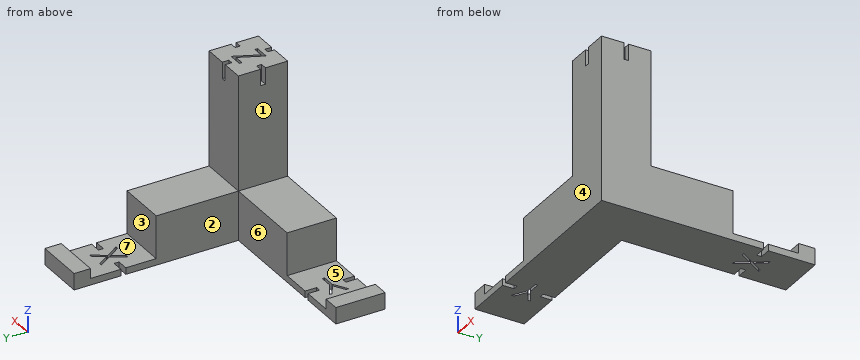
from build123d import *

# Parameters (mm, degrees)
CROQUIS2_W                = 25
CROQUIS2_H                = 15
SALIENTE_EXTRUIR1_DEPTH   = 15
CROQUIS2_W_2              = 15
CROQUIS2_H_2              = 25
SALIENTE_EXTRUIR1_2_DEPTH = 15
CROQUIS2_3_W              = 15
CROQUIS2_3_H              = 15
SALIENTE_EXTRUIR2_DEPTH   = 50
CROQUIS3_W                = 20
CROQUIS3_H                = 15
CROQUIS3_W_2              = 15
CROQUIS3_H_2              = 20
SALIENTE_EXTRUIR3_DEPTH   = 2
CROQUIS3_3_W              = 5
CROQUIS3_3_H              = 15
CROQUIS3_3_W_2            = 15
CROQUIS3_3_H_2            = 5
SALIENTE_EXTRUIR4_DEPTH   = 5
CROQUIS4_W                = 3.5
CROQUIS4_H                = 1.5
CROQUIS4_W_2              = 1.5
CROQUIS4_H_2              = 3.5
CORTAR_EXTRUIR1_DEPTH     = 15
CROQUIS5_W                = 1.5
CROQUIS5_H                = 2
CROQUIS5_W_2              = 2
CROQUIS5_H_2              = 1.5
CORTAR_EXTRUIR2_DEPTH     = 5


with BuildPart() as part:
    # Croquis2 → Saliente-Extruir1 (new body)
    with BuildSketch(Plane.XY):
        with Locations((-27.5, 7.5)):
            Rectangle(CROQUIS2_W, CROQUIS2_H)
    extrude(amount=SALIENTE_EXTRUIR1_DEPTH)



with BuildPart() as body_2:
    # Croquis2 → Saliente-Extruir1 2 (new body)
    with BuildSketch(Plane.XY):
        with Locations((-7.5, 27.5)):
            Rectangle(CROQUIS2_W_2, CROQUIS2_H_2)
    extrude(amount=SALIENTE_EXTRUIR1_2_DEPTH)


with BuildPart() as part_1:
    add(part.part)

    add(body_2.part)  # Saliente-Extruir2 merges body 2
    # Croquis2_3 → Saliente-Extruir2 (add)
    with BuildSketch(Plane.XY):
        with Locations((-7.5, 7.5)):
            Rectangle(CROQUIS2_3_W, CROQUIS2_3_H)
    extrude(amount=SALIENTE_EXTRUIR2_DEPTH)

    # Croquis3 → Saliente-Extruir3 (add)
    with BuildSketch(Plane.XY):
        with Locations((-50, 7.5)):
            Rectangle(CROQUIS3_W, CROQUIS3_H)
        with Locations((-7.5, 50)):
            Rectangle(CROQUIS3_W_2, CROQUIS3_H_2)
    extrude(amount=SALIENTE_EXTRUIR3_DEPTH)

    # Croquis3_3 → Saliente-Extruir4 (add)
    with BuildSketch(Plane.XY):
        with Locations((-62.5, 7.5)):
            Rectangle(CROQUIS3_3_W, CROQUIS3_3_H)
        with Locations((-7.5, 62.5)):
            Rectangle(CROQUIS3_3_W_2, CROQUIS3_3_H_2)
    extrude(amount=SALIENTE_EXTRUIR4_DEPTH)

    # Croquis4 → Cortar-Extruir1 (cut)
    with BuildSketch(Plane.XY.offset(2)):
        with Locations((-13.25, 50)):
            Rectangle(CROQUIS4_W, CROQUIS4_H)
        with Locations((-1.75, 50)):
            Rectangle(CROQUIS4_W, CROQUIS4_H)
        with Locations((-50, 13.25)):
            Rectangle(CROQUIS4_W_2, CROQUIS4_H_2)
        with Locations((-50, 1.75)):
            Rectangle(CROQUIS4_W_2, CROQUIS4_H_2)
        Polygon((-10.423076923, 54), (-9.594551282, 54), (-7.5, 50.727564103), (-5.405448718, 54), (-4.576923077, 54), (-7.084935897, 50.080128205), (-4.474358974, 46), (-5.302884615, 46), (-7.5, 49.432692308), (-9.697115385, 46), (-10.525641026, 46), (-7.913461538, 50.080128205), align=None)
        Polygon((-54, 10.423076923), (-54, 9.600961538), (-50.5625, 7.498397436), (-54, 5.399038462), (-54, 4.576923077), (-49.802884615, 7.141025641), (-46, 7.141025641), (-46, 7.858974359), (-49.802884615, 7.858974359), align=None)
    extrude(amount=-CORTAR_EXTRUIR1_DEPTH, mode=Mode.SUBTRACT)

    # Croquis5 → Cortar-Extruir2 (cut)
    with BuildSketch(Plane.XY.offset(50)):
        with Locations((-7.5, 14)):
            Rectangle(CROQUIS5_W, CROQUIS5_H)
        with Locations((-7.5, 1)):
            Rectangle(CROQUIS5_W, CROQUIS5_H)
        with Locations((-1, 7.5)):
            Rectangle(CROQUIS5_W_2, CROQUIS5_H_2)
        with Locations((-14, 7.5)):
            Rectangle(CROQUIS5_W_2, CROQUIS5_H_2)
        Polygon((-9.551282051, 10.679487179), (-9.551282051, 11.5), (-5.346153846, 11.5), (-8.701923077, 4.320512821), (-5.448717949, 4.320512821), (-5.448717949, 3.5), (-9.858974359, 3.5), (-6.503205128, 10.679487179), align=None)
    extrude(amount=-CORTAR_EXTRUIR2_DEPTH, mode=Mode.SUBTRACT)


solid = part_1.part
Could you check a few things on this model? Use its own coordinates, in mm. Face numbers are marked on the shaded views. A direction names the side the tool comes from. Give positions to 0.01 mm unless a question says otherwise; leave off trailing zeros. Order: outer loops, then holes, each group sorted by start corner. A loop starts at its lowest first (then second) coordinate and runs counter-clockwise, first axis right, second up.
1. Suppose I cut it at C-C (z = 14). Write out the boundary of the cut face in (x, y), plus the area to 3 significant figures.
Answers below:
outline: (-40, 0) - (0, 0) - (0, 40) - (-15, 40) - (-15, 15) - (-40, 15) - close
area: 975 mm2
2. I need wall thicknesses on L1, parallel to X at y = 36, z = 11; L2, parallel to X at y = 9.5, z = 12.5; L3, parallel to Z at x = -16.5, y = 6. Which ranges of each line are inside material? Lowest first, please.
Answers below:
L1: x = -15 to 0
L2: x = -40 to 0
L3: z = 0 to 15
3. Thinking about a two-plate mould opening in Y: for the marked faces 4, 5, 6 and 7, which applies, +Y half, -Y half, draft (parallel to the pull), parting line (faces both ways), or undercut?
Answers below:
face 4: -Y half
face 5: draft
face 6: +Y half
face 7: undercut
4. Suppose I cut it at B-B (y = 47.5). Write out the boundary of the cut face in (x, z), plus the area to 3 significant figures.
Answers below:
outline: (-15, 0) - (-9.57, 0) - (-9.57, 2) - (-15, 2) - close; (-8.74, 0) - (-6.26, 0) - (-6.26, 2) - (-8.74, 2) - close; (-5.43, 0) - (0, 0) - (0, 2) - (-5.43, 2) - close
area: 26.7 mm2
5. Suppose I cut it at D-D (y = 19). Write out the boundary of the cut face in (x, z).
Answers below:
outline: (-15, 0) - (0, 0) - (0, 15) - (-15, 15) - close
6. Which directions (+Z, -Z, +X, -X, +Y, -Y) give clear straight access to the entire face, cutting with the end or side of a thin tool? Please do the marked faces 1, 2 and 3.
Answers below:
face 1: +Z, -X, +Y, -Y
face 2: +Z, -Z, -X, +Y
face 3: +Z, +X, -X
7. Suppose I cut it at A-A (z = 46). Write out the boundary of the cut face in (x, y).
Answers below:
outline: (-15, 0) - (-8.25, 0) - (-8.25, 2) - (-6.75, 2) - (-6.75, 0) - (0, 0) - (0, 6.75) - (-2, 6.75) - (-2, 8.25) - (0, 8.25) - (0, 15) - (-6.75, 15) - (-6.75, 13) - (-8.25, 13) - (-8.25, 15) - (-15, 15) - (-15, 8.25) - (-13, 8.25) - (-13, 6.75) - (-15, 6.75) - close; hole (-9.86, 3.5) - (-5.45, 3.5) - (-5.45, 4.32) - (-8.7, 4.32) - (-5.35, 11.5) - (-9.55, 11.5) - (-9.55, 10.68) - (-6.5, 10.68) - close
8. For pin 1 (10 mm diameter, centred on x = -24.5, z = 37, fed in from +Y); pin 2 (0.8 mm diameter, centred on y = 50, z = 1.5, fed in from +X); pin 3 (5 mm diameter, centred on x = -15, y = 25.5, fed in from +Z); pin 4 (1.6 mm diameter, centred on y = 8, z = 48, fed in from -X), each with a flat end and sliding along its axis, tell me the tip position at first contact or that it passes through.
Answers below:
pin 1: passes through
pin 2: stops at x = -3.5
pin 3: stops at z = 15
pin 4: stops at x = -15
